```python
from build123d import *

# Parameters (mm, degrees)
SKETCH1_W           = 56
SKETCH1_H           = 34
BOSS_EXTRUDE1_DEPTH = 28
CUT_EXTRUDE1_DEPTH  = 12.75
CUT_EXTRUDE2_DEPTH  = 15.25
FILLET1_R           = 10
BOSS_EXTRUDE2_DEPTH = 10
SKETCH6_R           = 2.75
CUT_EXTRUDE3_DEPTH  = 34


with BuildPart() as part:
    # Sketch1 → Boss-Extrude1 (new body)
    with BuildSketch(Plane(origin=(0, 0, 0), x_dir=(1, 0, 0), z_dir=(0, 1, 0))):
        Rectangle(SKETCH1_W, SKETCH1_H)
    extrude(amount=BOSS_EXTRUDE1_DEPTH)

    # Sketch2 → Cut-Extrude1 (cut)
    with BuildSketch(Plane(origin=(0, 28, 0), x_dir=(1, 0, 0), z_dir=(0, 1, 0))):
        Polygon((-17, 7.982239485), (-8.35, -7), (8.35, -7), (17, 7.982239485), (17, 17), (-17, 17), align=None)
    extrude(amount=-CUT_EXTRUDE1_DEPTH, mode=Mode.SUBTRACT)

    # Sketch3 → Cut-Extrude2 (cut)
    with BuildSketch(Plane(origin=(0, 15.25, 0), x_dir=(1, 0, 0), z_dir=(0, 1, 0))):
        with BuildLine():
            Line((-14.375, 7.462624243), (-14.375, 17))
            Line((-14.375, 17), (14.375, 17))
            Line((14.375, 17), (14.375, 7.462624243))
            ThreePointArc((14.375, 7.462624243), (0, -6.912375757), (-14.375, 7.462624243))
        make_face()
    extrude(amount=-CUT_EXTRUDE2_DEPTH, mode=Mode.SUBTRACT)

    # Fillet1
    fillet1_edges = [part.edges().sort_by_distance(p)[0] for p in [
        (28, 14, 17),
        (-28, 14, 17),
    ]]
    fillet(fillet1_edges, radius=FILLET1_R)

    # Sketch5 → Boss-Extrude2 (add)
    with BuildSketch(Plane(origin=(0, 0, 7), x_dir=(-1, 0, 0), z_dir=(0, 0, -1))):
        with BuildLine():
            Line((18, 21), (18, 7))
            Line((18, 7), (21, 7))
            ThreePointArc((21, 7), (28, 14), (21, 21))
            Line((21, 21), (18, 21))
        make_face()
        with BuildLine():
            Line((-18, 7), (-21, 7))
            ThreePointArc((-21, 7), (-28, 14), (-21, 21))
            Line((-21, 21), (-18, 21))
            Line((-18, 21), (-18, 7))
        make_face()
    extrude(amount=-BOSS_EXTRUDE2_DEPTH)

    # Sketch6 → Cut-Extrude3 (cut)
    with BuildSketch(Plane.XY.offset(17)):
        with Locations((-21, 14)):
            Circle(SKETCH6_R)
        with Locations((21, 14)):
            Circle(SKETCH6_R)
    extrude(amount=-CUT_EXTRUDE3_DEPTH, mode=Mode.SUBTRACT)


solid = part.part
```
Design review of the part built by this model. Coordinates are the model's own, in mm. A direction names the side the tool comes from. Coordinates: 2 decimals unless noted, no trailing zeros. Order: outer loops, then holes, each group sorted by start corner. A loop starts at its lowest first (then second) coordinate and runs counter-clockwise, first axis right, second up. Notation, with made-up numbers: M 47,4.5 L 77,4.5 A22 ccw 77,40.5 Z; hole C 40,22.25 d2. An arc over 180 degrees is marked long. Answer as a JSON object with one key per item and string values. Group by question number.
1) Add section D-D, the plane z = 9.5. Write out the cut boundary in (x, y).
2) For pin 1 (5 mm diameter, centred on x = -21, y = 14, fed in from -Z); pin 2 (4 mm diameter, centred on x = 2, y = 24.5, fed in from -Z), all flat-tipped, find the tip position at first contact; note any pin that passes through.
3) Tool access review of faces 1 (the cylindrical face through (-28, 14, 14)), 2 (the flat face through (-14.375, 8, -12)), 3 (the cylindrical face through (26, 4, 13)), 4 (the flat face through (-17, 22, -13)): name each direction out of +Z, -Z, +X, -X, +Y, -Y from which nothing blocks a thin tool from reaching the whole face with its end or side.
4) Add section B-B, the plane x = 0. Write out the cut boundary in (y, z).
5) Mouldability with a two-part tool opening along Y and no side actions: class faces 5 (the flat face through (-21, 11, -17)), 6 (the flat face through (-0.4, 28, 7.3)), 7 (the cylindrical face through (-23.747, 14.121, 0.238)) as pulls with the +Y half, pulls with the -Y half, needs draft (parallel to the pull), parting line crosses it, or undercut.
6) Add section C-C, the plane y = 23.5. Write out the cut boundary in (x, z).
7) Wall thickness on L1, parallel to Y at x = 21, z = -5; L2, parallel to X at y = 20.25, z = -8; L3, parallel to X at y = 5.25, z = -9 (3 decimals): over which ranges is each line inside the solid? List them lowest first.
8) Add section A-A, the plane z = -9.5. Write out the cut boundary in (x, y) (3 decimals).
Computed values:
{
 "1": {"outline": "M -27.68,0 L 27.68,0 L 27.68,11.92 A7 ccw 27.68,16.08 L 27.68,28 L -27.68,28 L -27.68,16.08 A7 ccw -27.68,11.92 Z; hole C -21,14 d5.5; hole C 21,14 d5.5"},
 "2": {"pin 1": "passes through", "pin 2": "stops at z = 7"},
 "3": {"face 1": "+Z, -X", "face 2": "-Z, +Y, -Y", "face 3": "+Z, +X, -Y", "face 4": "-Z, +Y"},
 "4": {"outline": "M 0,6.91 L 15.25,6.91 L 15.25,7 L 28,7 L 28,17 L 0,17 Z"},
 "5": {"face 5": "needs draft", "face 6": "pulls with the +Y half", "face 7": "undercut"},
 "6": {"outline": "M -28,-17 L -17,-17 L -17,-7.98 L -8.35,7 L 8.35,7 L 17,-7.98 L 17,-17 L 28,-17 L 28,7 A10 ccw 18,17 L -18,17 A10 ccw -28,7 Z"},
 "7": {"L1": "y = 0 to 11.25, 16.75 to 28", "L2": "x = -28 to -17, 17 to 28", "L3": "x = -28 to -14.375, 14.375 to 28"},
 "8": {"outline": "M -28,0 L -14.375,0 L -14.375,15.25 L -17,15.25 L -17,28 L -28,28 Z; M 14.375,0 L 28,0 L 28,28 L 17,28 L 17,15.25 L 14.375,15.25 Z; hole C -21,14 d5.5; hole C 21,14 d5.5"}
}
